Source: CAD feature listing. Evaluate the final solid. Frame: model axes, mm. Face numbers are marked on the shaded views. A direction names the side the tool comes from. Give positions to 0.01 mm unless a question says otherwise; leave off trailing zeros. Order: outer loops, then holes, each group sorted by start corner. A loop starts at its lowest first (then second) coordinate and runs counter-clockwise, first axis right, second up. Notation, with made-up numbers: (84.5, -5.5) - (140.5, -5.5) arc R17 ccw to (140.5, 7.5) - close; hole circle Ø8 at (67.5, 34). An arc over 180 degrees is marked (long way). Answer as CSV lines item,"result".
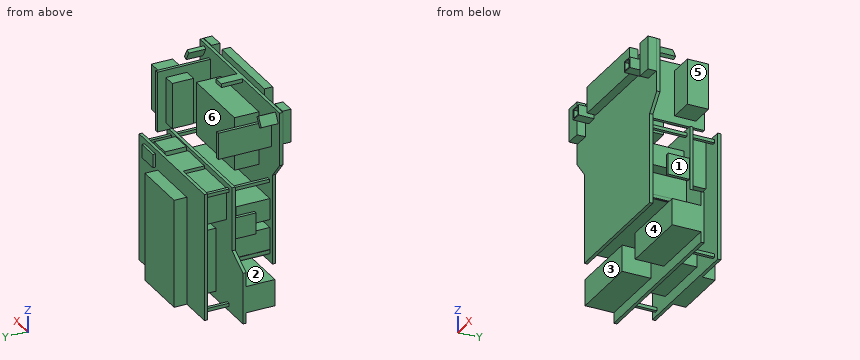
```python
from build123d import *

# Parameters (mm, degrees)
BOSS_EXTRUDE1_DEPTH       = 3
SKETCH2_W                 = 3.05
SKETCH2_H                 = 3.05
BOSS_EXTRUDE2_DEPTH       = 35
SKETCH3_W                 = 120
SKETCH3_H                 = 120
BOSS_EXTRUDE3_DEPTH       = 3
SKETCH4_W                 = 3.05
SKETCH4_H                 = 3.05
BOSS_EXTRUDE4_DEPTH       = 23
SKETCH6_W                 = 120
SKETCH6_H                 = 120
BOSS_EXTRUDE5_DEPTH       = 3
SKETCH7_W                 = 68
SKETCH7_H                 = 25
BOSS_EXTRUDE6_DEPTH       = 27
SKETCH9_W                 = 58
SKETCH9_H                 = 60
SKETCH9_W_2               = 20
SKETCH9_H_2               = 45
SKETCH9_W_3               = 50
SKETCH9_H_3               = 30
BOSS_EXTRUDE7_DEPTH       = 20
SKETCH10_W                = 53.46
SKETCH10_H                = 101.85
BOSS_EXTRUDE8_DEPTH       = 12
SKETCH11_W                = 110
SKETCH11_H                = 20
BOSS_EXTRUDE9_DEPTH       = 32
SKETCH12_W                = 110
SKETCH12_H                = 25
BOSS_EXTRUDE10_DEPTH      = 34
SKETCH13_W                = 20
SKETCH13_H                = 12.6
BOSS_EXTRUDE11_DEPTH      = 2.5
SKETCH14_W                = 3
SKETCH14_H                = 20
BOSS_EXTRUDE12_DEPTH      = 20
BOSS_EXTRUDE13_DEPTH      = 16
SKETCH16_W                = 3
SKETCH16_H                = 57
SKETCH16_H_2              = 25
BOSS_EXTRUDE14_DEPTH      = 50
BOSS_EXTRUDE15_DEPTH      = 23.4
BOSS_EXTRUDE15_DEPTH_BACK = 14.9
SKETCH17_W                = 43
SKETCH17_H                = 20
SKETCH18_W                = 78
SKETCH18_H                = 25
SKETCH18_W_2              = 14.4
SKETCH18_H_2              = 31.3
BOSS_EXTRUDE16_DEPTH      = 8
SKETCH20_W                = 10
SKETCH20_H                = 10
BOSS_EXTRUDE18_DEPTH      = 14.56
SKETCH21_W                = 8
SKETCH21_H                = 8
CUT_EXTRUDE1_DEPTH        = 5
SKETCH22_W                = 10
SKETCH22_H                = 3.5
BOSS_EXTRUDE19_DEPTH      = 20
SKETCH23_W                = 30
SKETCH23_H                = 3
BOSS_EXTRUDE20_DEPTH      = 20
SKETCH24_W                = 70
SKETCH24_H                = 50
BOSS_EXTRUDE21_DEPTH      = 23


with BuildPart() as part:
    # Sketch1 → Boss-Extrude1 (new body)
    with BuildSketch(Plane(origin=(0, 0, 0), x_dir=(1, 0, 0), z_dir=(0, 1, 0))):
        Polygon((-73, -25), (-60, -9.801315846), (-60, 75), (60, 75), (60, -9.801315846), (73, -25), (73, -75), (60, -75), (-60, -75), (-73, -75), align=None)
    extrude(amount=BOSS_EXTRUDE1_DEPTH)

    # Sketch2 → Boss-Extrude2 (add)
    with BuildSketch(Plane(origin=(0, 3, 0), x_dir=(1, 0, 0), z_dir=(0, 1, 0))):
        with Locations((-53, -1.81)):
            Rectangle(SKETCH2_W, SKETCH2_H)
        with Locations((53, -1.81)):
            Rectangle(SKETCH2_W, SKETCH2_H)
        with Locations((54, 65)):
            Rectangle(SKETCH2_W, SKETCH2_H)
        with Locations((-54, 65)):
            Rectangle(SKETCH2_W, SKETCH2_H)
    extrude(amount=BOSS_EXTRUDE2_DEPTH)

    # Sketch3 → Boss-Extrude3 (add)
    with BuildSketch(Plane(origin=(0, 38, 0), x_dir=(1, 0, 0), z_dir=(0, 1, 0))):
        Polygon((-80, 64.780305915), (-60, 52.99), (-60, 112.99), (-80, 112.99), align=None)
        with Locations((0, 52.99)):
            Rectangle(SKETCH3_W, SKETCH3_H)
        Polygon((60, 112.99), (60, 52.99), (80, 64.780305915), (80, 112.99), align=None)
    extrude(amount=BOSS_EXTRUDE3_DEPTH)

    # Sketch4 → Boss-Extrude4 (add)
    with BuildSketch(Plane(origin=(0, 41, 0), x_dir=(1, 0, 0), z_dir=(0, 1, 0))):
        with Locations((-53, -1.81)):
            Rectangle(SKETCH4_W, SKETCH4_H)
        with Locations((-53, 106.99)):
            Rectangle(SKETCH4_W, SKETCH4_H)
        with Locations((53, -1.81)):
            Rectangle(SKETCH4_W, SKETCH4_H)
        with Locations((53, 106.99)):
            Rectangle(SKETCH4_W, SKETCH4_H)
    extrude(amount=BOSS_EXTRUDE4_DEPTH)

    # Sketch6 → Boss-Extrude5 (add)
    with BuildSketch(Plane(origin=(0, 64, 0), x_dir=(1, 0, 0), z_dir=(0, 1, 0))):
        with Locations((0, 52.99)):
            Rectangle(SKETCH6_W, SKETCH6_H)
    extrude(amount=BOSS_EXTRUDE5_DEPTH)

    # Sketch7 → Boss-Extrude6 (add)
    with BuildSketch(Plane.XZ.offset(-38)):
        with Locations((-46, -90.53)):
            Rectangle(SKETCH7_W, SKETCH7_H)
        with Locations((46, -90.53)):
            Rectangle(SKETCH7_W, SKETCH7_H)
    extrude(amount=BOSS_EXTRUDE6_DEPTH)

    # Sketch9 → Boss-Extrude7 (add)
    with BuildSketch(Plane(origin=(0, 41, 0), x_dir=(1, 0, 0), z_dir=(0, 1, 0))):
        with Locations((-1.05, 75.88)):
            Rectangle(SKETCH9_W, SKETCH9_H)
        with Locations((34, 16.79)):
            Rectangle(SKETCH9_W_2, SKETCH9_H_2)
        with Locations((-24.66, 13.16)):
            Rectangle(SKETCH9_W_3, SKETCH9_H_3)
    extrude(amount=BOSS_EXTRUDE7_DEPTH)

    # Sketch10 → Boss-Extrude8 (add)
    with BuildSketch(Plane(origin=(0, 67, 0), x_dir=(1, 0, 0), z_dir=(0, 1, 0))):
        with Locations((-0.81, 62.065)):
            Rectangle(SKETCH10_W, SKETCH10_H)
    extrude(amount=BOSS_EXTRUDE8_DEPTH)

    # Sketch11 → Boss-Extrude9 (add)
    with BuildSketch(Plane(origin=(0, 3, 0), x_dir=(1, 0, 0), z_dir=(0, 1, 0))):
        with Locations((0, 25)):
            Rectangle(SKETCH11_W, SKETCH11_H)
    extrude(amount=BOSS_EXTRUDE9_DEPTH)

    # Sketch12 → Boss-Extrude10 (add)
    with BuildSketch(Plane(origin=(0, 3, 0), x_dir=(1, 0, 0), z_dir=(0, 1, 0))):
        with Locations((0, 55)):
            Rectangle(SKETCH12_W, SKETCH12_H)
    extrude(amount=BOSS_EXTRUDE10_DEPTH)

    # Sketch13 → Boss-Extrude11 (add)
    with BuildSketch(Plane(origin=(0, 67, 0), x_dir=(1, 0, 0), z_dir=(0, 1, 0))):
        with Locations((40, 3.91)):
            Rectangle(SKETCH13_W, SKETCH13_H)
    extrude(amount=BOSS_EXTRUDE11_DEPTH)

    # Sketch14 → Boss-Extrude12 (add)
    with BuildSketch(Plane(origin=(0, 38, 0), x_dir=(1, 0, 0), z_dir=(0, 1, 0))):
        with Locations((57.5, 32.99)):
            Rectangle(SKETCH14_W, SKETCH14_H)
        with Locations((-57.5, 32.99)):
            Rectangle(SKETCH14_W, SKETCH14_H)
    extrude(amount=-BOSS_EXTRUDE12_DEPTH)

    # Sketch15 → Boss-Extrude13 (add)
    with BuildSketch(Plane(origin=(0, 3, 0), x_dir=(1, 0, 0), z_dir=(0, 1, 0))):
        Polygon((65.5, -72.5), (62.468911087, -70.75), (67.468911087, -62.089745962), (70.5, -63.839745962), align=None)
        Polygon((-70.5, -63.839745962), (-65.5, -72.5), (-62.468911087, -70.75), (-67.468911087, -62.089745962), align=None)
    extrude(amount=BOSS_EXTRUDE13_DEPTH)

    # Sketch16 → Boss-Extrude14 (add)
    with BuildSketch(Plane(origin=(0, 3, 0), x_dir=(1, 0, 0), z_dir=(0, 1, 0))):
        with Locations((55.5, -36.6)):
            Rectangle(SKETCH16_W, SKETCH16_H)
        with Locations((-56.5, -48.5)):
            Rectangle(SKETCH16_W, SKETCH16_H_2)
    extrude(amount=BOSS_EXTRUDE14_DEPTH)

    # Sketch17 → Boss-Extrude15 (add, two sides: drawn at the far end of the back side and taken through both)
    with BuildSketch(Plane(origin=(57, 0, 0), x_dir=(0, 0, -1), z_dir=(1, 0, 0)).offset(-BOSS_EXTRUDE15_DEPTH_BACK)):
        with Locations((-36.6, 35)):
            Rectangle(SKETCH17_W, SKETCH17_H)
    extrude(amount=BOSS_EXTRUDE15_DEPTH + BOSS_EXTRUDE15_DEPTH_BACK)

    # Sketch18 → Boss-Extrude16 (add)
    with BuildSketch(Plane.XZ):
        with Locations((0, 68.5)):
            Rectangle(SKETCH18_W, SKETCH18_H)
        with Locations((-65, 60.1)):
            Rectangle(SKETCH18_W_2, SKETCH18_H_2)
        with Locations((65, 60.1)):
            Rectangle(SKETCH18_W_2, SKETCH18_H_2)
    extrude(amount=BOSS_EXTRUDE16_DEPTH)

    # Sketch20 → Boss-Extrude18 (add)
    with BuildSketch(Plane.XZ):
        with Locations((-46.89, 59)):
            Rectangle(SKETCH20_W, SKETCH20_H)
        with Locations((46.89, 59)):
            Rectangle(SKETCH20_W, SKETCH20_H)
    extrude(amount=BOSS_EXTRUDE18_DEPTH)

    # Sketch21 → Cut-Extrude1 (cut)
    with BuildSketch(Plane.XZ.offset(14.56)):
        with Locations((46.89, 59)):
            Rectangle(SKETCH21_W, SKETCH21_H)
        with Locations((-46.89, 59)):
            Rectangle(SKETCH21_W, SKETCH21_H)
    extrude(amount=-CUT_EXTRUDE1_DEPTH, mode=Mode.SUBTRACT)

    # Sketch22 → Boss-Extrude19 (add)
    with BuildSketch(Plane(origin=(0, 3, 0), x_dir=(1, 0, 0), z_dir=(0, 1, 0))):
        with Locations((0, -73.25)):
            Rectangle(SKETCH22_W, SKETCH22_H)
    extrude(amount=BOSS_EXTRUDE19_DEPTH)

    # Sketch23 → Boss-Extrude20 (add)
    with BuildSketch(Plane.XZ.offset(-64)):
        with Locations((0, 5.51)):
            Rectangle(SKETCH23_W, SKETCH23_H)
    extrude(amount=BOSS_EXTRUDE20_DEPTH)

    # Sketch24 → Boss-Extrude21 (add)
    with BuildSketch(Plane(origin=(0, 3, 0), x_dir=(1, 0, 0), z_dir=(0, 1, 0))):
        with Locations((0, -33)):
            Rectangle(SKETCH24_W, SKETCH24_H)
    extrude(amount=BOSS_EXTRUDE21_DEPTH)


solid = part.part
```
(1) Cut plane C-C (z = -3). Return loops of the section in (x, y), then the cut area to 3 significant figures.
Completed:
outline,"(-60, 0) - (60, 0) - (60, 3) - (-60, 3) - close; (-60, 38) - (60, 38) - (60, 41) - (44, 41) - (44, 61) - (24, 61) - (24, 41) - (0.34, 41) - (0.34, 61) - (-49.66, 61) - (-49.66, 41) - (-60, 41) - close; (-60, 64) - (60, 64) - (60, 67) - (50, 67) - (50, 69.5) - (30, 69.5) - (30, 67) - (-60, 67) - close"
area,"2,530 mm²"
(2) Contact query for flat-ended pins moving along their axis: pin 1 (3 mm diameter, centred on x = 2, y = 10.5, fed in from -Z); pin 2 (6 mm diameter, centred on x = 46, z = 31.5, fed in from -Y); pin 3 (1.5 mm diameter, centred on x = 56, y = 30, fed in from -Z). Output: stop coordinate, or through.
Completed:
pin 1,"z = -67.5"
pin 2,"y = 0"
pin 3,"z = -103.03"
(3) Cut plane B-B (y = 56). Give the number of separate pieces and of enclosed holes in the cut face, then the cut area to 3 significant figures.
Completed:
separate pieces,"8"
enclosed holes,"0"
area,"6,010 mm²"
(4) Access query for the marked faces 1, 2 and 3. Directions: +Z, -Z, +X, -X, +Y, -Y. A direction counts if a zero-diameter tool reaches every point of the face in a straight line with its end or side. Return the directions, or none.
Completed:
face 1,"+X"
face 2,"+X, -X, -Y"
face 3,"-Z, +X, -X, -Y"
(5) Ray query, line 1 (Y direction, x = 53, z = -34.5); line 2 (Y direction, x = -46, z = -57); line 3 (Z direction, x = -20, y = 28). Return the intervals inside material, ascending. Write a range as from..to.
Completed:
line 1,"0..35, 38..41, 64..67"
line 2,"0..37, 38..41, 64..67"
line 3,"-103.03..-78.03, -67.5..-42.5, -35..-15"
(6) Mould query, pull axis X, two halves, no side actions, for the marked faces 4, 5 and 6. Classes: released by +X, released by -X, zero draft, split by the parting line, or undercut.
Completed:
face 4,"zero draft"
face 5,"released by +X"
face 6,"undercut"
(7) Cut plane A-A (z = -81). Return loops of the section in (x, y).
Completed:
outline,"(-80, 11) - (-12, 11) - (-12, 38) - (12, 38) - (12, 11) - (80, 11) - (80, 41) - (27.95, 41) - (27.95, 61) - (-30.05, 61) - (-30.05, 41) - (-80, 41) - close; (-60, 64) - (60, 64) - (60, 67) - (25.92, 67) - (25.92, 79) - (-27.54, 79) - (-27.54, 67) - (-60, 67) - close"
